from build123d import *

# Parameters (mm, degrees)
BOSS_EXTRUDE1_DEPTH = 4
SKETCH2_R           = 1.5
SKETCH2_R_2         = 4.8
SKETCH2_R_3         = 2
CUT_EXTRUDE1_DEPTH  = 10
SKETCH3_W           = 7
SKETCH3_H           = 22.146248503
SKETCH3_W_2         = 7.418721668
SKETCH3_H_2         = 10.140288501
BOSS_EXTRUDE2_DEPTH = 6.2
SKETCH4_R           = 1
CUT_EXTRUDE2_DEPTH  = 70
SKETCH5_R           = 1.5
CUT_EXTRUDE3_DEPTH  = 3
CUT_EXTRUDE3_DRAFT  = -32


with BuildPart() as part:
    # Sketch1 → Boss-Extrude1 (new body)
    with BuildSketch(Plane.XY):
        with BuildLine():
            Line((18, 32), (18, 39))
            ThreePointArc((18, 39), (17.707106781, 39.707106781), (17, 40))
            Line((17, 40), (14, 40))
            ThreePointArc((14, 40), (13.292893219, 39.707106781), (13, 39))
            Line((13, 39), (13, 33))
            ThreePointArc((13, 33), (12.707106781, 32.292893219), (12, 32))
            Line((12, 32), (-12, 32))
            ThreePointArc((-12, 32), (-12.707106781, 32.292893219), (-13, 33))
            Line((-13, 33), (-13, 39))
            ThreePointArc((-13, 39), (-13.292893219, 39.707106781), (-14, 40))
            Line((-14, 40), (-17, 40))
            ThreePointArc((-17, 40), (-17.707106781, 39.707106781), (-18, 39))
            Line((-18, 39), (-18, 32))
            Line((-18, 32), (-18, -32))
            Line((-18, -32), (18, -32))
            Line((18, -32), (18, 32))
        make_face()
    extrude(amount=BOSS_EXTRUDE1_DEPTH)

    # Sketch2 → Cut-Extrude1 (cut)
    with BuildSketch(Plane.XY.offset(4)):
        with Locations((15.5, 29.744145571)):
            Circle(SKETCH2_R)
        with Locations((-14, 27)):
            Circle(SKETCH2_R)
        with Locations((4.475, 10.927702889)):
            Circle(SKETCH2_R_2)
        with Locations((-14, -2.442942894)):
            Circle(SKETCH2_R)
        with Locations((14, -9.442942894)):
            Circle(SKETCH2_R)
        with Locations((-4.475, -22.442942894)):
            Circle(SKETCH2_R_2)
        with Locations((13.025, -27.642942894)):
            Circle(SKETCH2_R_3)
        with Locations((-14, -22.442942894)):
            Circle(SKETCH2_R_3)
        with Locations((-13.025, 16.127702889)):
            Circle(SKETCH2_R_3)
        with Locations((15.5, 37.5)):
            Circle(SKETCH2_R)
        with Locations((-15.5, 37.5)):
            Circle(SKETCH2_R)
    extrude(amount=-CUT_EXTRUDE1_DEPTH, mode=Mode.SUBTRACT)

    # Sketch3 → Boss-Extrude2 (add)
    with BuildSketch(Plane.XY.offset(4)):
        with Locations((0.209360834, -5.740885149)):
            Rectangle(SKETCH3_W, SKETCH3_H)
        with Locations((0, 22.037818849)):
            Rectangle(SKETCH3_W_2, SKETCH3_H_2)
    extrude(amount=BOSS_EXTRUDE2_DEPTH)

    # Sketch4 → Cut-Extrude2 (cut)
    with BuildSketch(Plane.XZ.offset(16.8140094)):
        with Locations((0, 7.165)):
            Circle(SKETCH4_R)
    extrude(amount=-CUT_EXTRUDE2_DEPTH, mode=Mode.SUBTRACT)


with BuildPart() as cut_extrude3_tool:
    # Sketch5 → Cut-Extrude3 (with draft: the straight prism first)
    with BuildSketch(Plane(origin=(0, 5.332239103, 0), x_dir=(-1, 0, 0), z_dir=(0, 1, 0))):
        with Locations((0, 7.165)):
            Circle(SKETCH5_R)
    extrude(amount=-CUT_EXTRUDE3_DEPTH)
    # Cut-Extrude3: the draft: its side faces are tilted about the plane it starts from
    cut_extrude3_sides = [cut_extrude3_tool.faces().sort_by_distance(p)[0] for p in [
        (1.5, 3.832239103, 7.165),
    ]]
    draft(cut_extrude3_sides, Plane(origin=(0, 5.332239103, 0), x_dir=(-1, 0, 0), z_dir=(0, 1, 0)), CUT_EXTRUDE3_DRAFT)


with BuildPart() as part_1:
    add(part.part)

    # Cut-Extrude3: cut by cut_extrude3_tool
    add(cut_extrude3_tool.part, mode=Mode.SUBTRACT)


solid = part_1.part
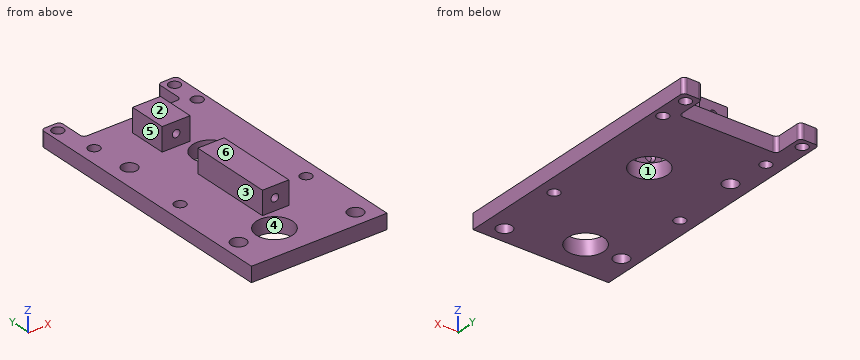
Part model, mm, in its own coordinate system. Face numbers are marked on the shaded views. A direction names the side the tool comes from. Round coordinates to 2 decimals unless told otherwise and drop trailing zeros. Write each loop counter-clockwise with the first axis right and the second up, starting at its lowest first coordinate (ties: lowest second). Pieces come first, ordered by that corner, then holes. Notation, with made-up numbers: (-2, 63.5) - (47, 63.5) arc R13 cw to (47, 75.5) - close; hole circle Ø6 at (39, -19). An arc over 180 degrees is marked (long way). Use CSV: the item, a comma, the result in double quotes.
Item 1: Wall check: L1, parallel to Z at x = 0, y = 22 (3 decimals); L2, parallel to Y at x = 4.5, z = 3.5; L3, parallel to Z at x = -11.5, y = -4. Give the ranges that are in metal, low to high.
Results list:
L1,"z = 0 to 6.165, 8.165 to 10.2"
L2,"y = -32 to 6.13, 15.73 to 32"
L3,"z = 0 to 4"
Item 2: Tool access for the marked faces 5 and 6: list every direction of +Z, -Z, +X, -X, +Y, -Y with a clear straight run to the whole face (end or side of a thin tool).
Results list:
face 5,"+Z, -X, +Y, -Y"
face 6,"+Z, +X, -X, +Y, -Y"
Item 3: Flat gauge pins, fed straight in: P1, Ø5, axis at x = -14, y = -22.44, coming from the +Z side; P2, Ø2.5, axis at x = -14, y = -2.44, coming from the -Z side; P3, Ø1, axis at y = 20.5, z = 9, coming from the -X side; P4, Ø1.9, axis at x = -1, z = 8, coming from the +Y side. Where does each tip first touch, or does it go through?
Results list:
P1,"stops at z = 4"
P2,"passes through"
P3,"stops at x = -3.71"
P4,"stops at y = 27.11"
Item 4: Slice it at A-A, the plane y = 37.5. Write the cut outline in (x, z), then the cut area to 3 significant figures.
Results list:
outline,"(-18, 0) - (-17, 0) - (-17, 4) - (-18, 4) - close; (-14, 0) - (-13, 0) - (-13, 4) - (-14, 4) - close; (13, 0) - (14, 0) - (14, 4) - (13, 4) - close; (17, 0) - (18, 0) - (18, 4) - (17, 4) - close"
area,"16.0 mm²"
Item 5: Slice it at B-B, the plane z = 2.25. Count the separate pieces of the cut face and the enclosed holes in it, then the cut area to 3 significant figures.
Results list:
separate pieces,"1"
enclosed holes,"11"
area,"2,160 mm²"
Item 6: Pull direction X, two halves, no side cores. Call the marked faces 1, 2, 3 and 4: pulls with the +X half, pulls with the -X half, needs draft (parallel to the pull), parting line crosses it, or undercut.
Results list:
face 1,"undercut"
face 2,"needs draft"
face 3,"pulls with the -X half"
face 4,"undercut"
